```python
from build123d import *

# Parameters (mm, degrees)
F0_R     = 39.324238
F0_R_2   = 21.491719
F1_DEPTH = 18.288
F2_DEPTH = 25.4
F3_R     = 5.08


with BuildPart() as f1:
    # F0 (on Top) → F1 (new body)
    with BuildSketch(Plane.XY):
        with Locations((3.718213, 0)):
            Circle(F0_R)
        with Locations((3.718213, 0)):
            Circle(F0_R_2, mode=Mode.SUBTRACT)
    extrude(amount=F1_DEPTH)

    # F0 (on Top) → F2 (join)
    with BuildSketch(Plane.XY):
        with Locations((3.718213, 0)):
            Circle(F0_R)
        with Locations((3.718213, 0)):
            Circle(F0_R_2, mode=Mode.SUBTRACT)
    extrude(amount=F2_DEPTH)

    # F3
    f3_edges = [f1.edges().sort_by_distance(p)[0] for p in [
        (-35.606025, 0, 25.4),
        (-17.773505, 0, 25.4),
    ]]
    fillet(f3_edges, radius=F3_R)


solid = f1.part
```
The listing builds one solid part. Answer for the finished solid, in the listing's coordinates (mm). Coordinates: 2 decimals unless noted, no trailing zeros. Order: outer loops, then holes, each group sorted by start corner. A loop starts at its lowest first (then second) coordinate and runs counter-clockwise, first axis right, second up. Notation, with made-up numbers: M 87.5,-10.75 L 111.5,-10.75 A7 ccw 111.5,0.25 Z; hole C 86,82.5 d9. An arc over 180 degrees is marked long. Answer as a JSON object with one key per item and string values. Group by question number.
1. Determine the mould class of faces 1 (the cylindrical face through (24.217, 6.456, 10.018)), 2 (the cylindrical face through (-27.488, -23.928, 10.018)), 3 (the flat face through (21.31, -20.13, 25.4)) for opening direction X: released by +X, released by -X, zero draft, split by the parting line, or undercut.
2. Flat-ended cylindrical pins translate along their axes: P1, Ø2, axis at y = 5.5, z = 16.5, coming from the -X side; P2, Ø1.5, axis at x = 22.5, z = 17, coming from the +Y side; P3, Ø4, axis at x = -4.5, z = 4.5, coming from the -Y side. Find the tip coordinate at first contact, or state that the pin passes through.
3. Section A-A on y = 0 is taken. Write down the section's boundary in (x, z).
4. Section C-C on z = 22.75 is taken. Write down the section's boundary in (x, y), then the cut area to 3 significant figures.
5. Section B-B on z = 15.75 is taken. Write down the section's boundary in (x, y), then the cut area to 3 significant figures.
6. Straight lines are drawn through the part: line 1 (Y direction, x = 2, z = 6.5); line 2 (X direction, y = 2, z = 11); line 3 (Y direction, x = -5.5, z = 21.5). For each, find the intervals that lie inside material, in ascending order.
Values follow:
{
 "1": {"face 1": "undercut", "face 2": "split by the parting line", "face 3": "zero draft"},
 "2": {"P1": "x = -35.35", "P2": "y = 34.95", "P3": "y = -38.83"},
 "3": {"outline": "M -35.61,0 L -17.77,0 L -17.77,20.32 A5.08 ccw -22.85,25.4 L -30.53,25.4 A5.08 ccw -35.61,20.32 Z; M 25.21,0 L 43.04,0 L 43.04,20.32 A5.08 ccw 37.96,25.4 L 30.29,25.4 A5.08 ccw 25.21,20.32 Z"},
 "4": {"outline": "C 3.72,0 d77.41; hole C 3.72,0 d44.22", "area": "3,170 mm2"},
 "5": {"outline": "C 3.72,0 d78.65; hole C 3.72,0 d42.98", "area": "3,410 mm2"},
 "6": {"line 1": "-39.29 to -21.42, 21.42 to 39.29", "line 2": "-35.56 to -17.68, 25.12 to 42.99", "line 3": "-38.09 to -19.57, 19.57 to 38.09"}
}
